CAD build for the part. Positions are in the model's coordinates, mm. A direction names the side the tool comes from. Coordinates: 2 decimals unless noted, no trailing zeros. Order: outer loops, then holes, each group sorted by start corner. A loop starts at its lowest first (then second) coordinate and runs counter-clockwise, first axis right, second up. Notation, with made-up numbers: (77.25, 0) - (130.25, 0) arc R21 cw to (130.25, 4) - close; hole circle Ø2 at (63.25, -33). An arc over 180 degrees is marked (long way). Write each question's results on one line, items separated by ' | '. Start each with the question number.
Q1. Band-saw the part on B-B, the plane z = 28.5. Write the cut outline in (x, y).
Q2. Band-saw the part on A-A, the plane x = -49. Write the cut outline in (y, z).
Q3. Band-saw the part on D-D, the plane z = -6. Write the cut outline in (x, y), then the cut area to 3 significant figures.
Q4. Wall check: probe 1 along X at (y, z) = (-11.5, -30.5); probe 2 along X at (y, z) = (40.5, 32.5); probe 3 along Z at (x, y) = (-5.5, 59). Give the ranges that are in metal, low to high.
Q5. Pin check, flat tips, straight feed: P1, Ø10, axis at x = 57.5, y = -5.5, coming from the +Z side; P2, Ø7.5, axis at y = 5, z = -31, coming from the +X side; P3, Ø12, axis at x = -0.5, y = 25.5, coming from the +Z side. Stop position of each tip, or through.
Q6. Band-saw the part on C-C, the plane z = 14. Write the cut outline in (x, y), then the cut area to 3 significant figures.
Q7. Which spindle directions (+Z, -Z, +X, -X, +Y, -Y) get a long thin tool onto all of the face, cutting with end or side? Do faces 1 (the flat face through (29.781, 1, -28)), 2 (the flat face through (46.28, 1.3, 44.5)), 3 (the flat face through (28.229, 1.301, 21.824)). Say none if no direction does.
Q8. Pull direction Z, two halves, no side cores. Call faces 4 (the flat face through (-46.28, 1.3, 44.5)), 5 (the flat face through (17.946, 1.301, -33.956)), 6 (the flat face through (1, 72.644, 3)), 7 (the flat face through (12.2, 1.3, 52.7)): released by +Z, released by -Z, zero draft, split by the parting line, or undercut.
```python
from build123d import *

# Parameters (mm, degrees)
F1_DEPTH      = 68.072
F1_DEPTH_BACK = 72.644


with BuildPart() as f1:
    # F0 (on Front) → F1 (new body, two sides)
    with BuildSketch(Plane.XZ) as f1_sk:
        with BuildLine():
            Line((-43.8699675724, 4.9395202659), (-26.3915906821, 9.9711745287))
            ThreePointArc((-26.3915906821, 9.9711745287), (-27.2085319986, 17.0209655839), (-26.1747674174, 24.042238818))
            Line((-26.1747674174, 24.042238818), (-30.3419636079, 19.5435739099))
            Line((-30.3419636079, 19.5435739099), (-43.8699675724, 4.9395202659))
        make_face()
        with BuildLine():
            ThreePointArc((-9.5438323287, 42.0849398232), (-15.4092627723, 39.0301381471), (-20.3645734785, 34.6506423572))
            Line((-20.3645734785, 34.6506423572), (-7.1865939535, 29.6427810635))
            Line((-7.1865939535, 29.6427810635), (-7.1865939535, 32.6668713242))
            Line((-7.1865939535, 32.6668713242), (-9.5438323287, 42.0849398232))
        make_face()
        with BuildLine():
            Line((0, -36.5192646342), (0, -10.610057041))
            ThreePointArc((0, -10.610057041), (-16.7339710743, -4.8564916944), (-26.3915906821, 9.9711745287))
            Line((-26.3915906821, 9.9711745287), (-43.8699675724, 4.9395202659))
            Line((-43.8699675724, 4.9395202659), (-30.3419636079, 19.5435739099))
            Line((-30.3419636079, 19.5435739099), (-65.5041635036, 38.4049154818))
            Line((-65.5041635036, 38.4049154818), (-60.6228390417, 21.448736815))
            Line((-60.6228390417, 21.448736815), (-43.8699675724, -2.8352683876))
            Line((-43.8699675724, -2.8352683876), (-40.2366704703, -3.5186973045))
            Line((-40.2366704703, -3.5186973045), (-43.8699675724, -9.0736041914))
            Line((-43.8699675724, -9.0736041914), (-37.7853512764, -20.751086995))
            Line((-37.7853512764, -20.751086995), (-29.7805646327, -25.9867765768))
            Line((-29.7805646327, -25.9867765768), (-29.7805646327, -29.878012836))
            Line((-29.7805646327, -29.878012836), (-25.9352512658, -32.3328636587))
            Line((-25.9352512658, -32.3328636587), (-21.6632075608, -32.3328636587))
            Line((-21.6632075608, -32.3328636587), (-14.1229508445, -35.6245934963))
            Line((-14.1229508445, -35.6245934963), (-14.1229508445, -25.9867765768))
            Line((-14.1229508445, -25.9867765768), (-8.1736836948, -29.878012836))
            Line((-8.1736836948, -29.878012836), (-3.4166643449, -34.2845275061))
            Line((-3.4166643449, -34.2845275061), (0, -36.5192646342))
        make_face()
        Polygon((0, 26.9117504358), (-7.1865939535, 29.6427810635), (-7.1865939535, 21.905059882), align=None)
        with BuildLine():
            Line((-7.1865939535, 42.5278679195), (-7.293939468, 42.8177008727))
            ThreePointArc((-7.293939468, 42.8177008727), (-8.4268543632, 42.4757869761), (-9.5438323287, 42.0849398232))
            Line((-9.5438323287, 42.0849398232), (-7.1865939535, 32.6668713242))
            Line((-7.1865939535, 32.6668713242), (-7.1865939535, 42.5278679195))
        make_face()
        with BuildLine():
            ThreePointArc((-20.3645734785, 34.6506423572), (-23.8665481201, 29.673348875), (-26.1747674174, 24.042238818))
            Line((-26.1747674174, 24.042238818), (-14.7990193218, 16.6017049924))
            Line((-14.7990193218, 16.6017049924), (-7.1865939535, 21.905059882))
            Line((-7.1865939535, 21.905059882), (-7.1865939535, 29.6427810635))
            Line((-7.1865939535, 29.6427810635), (-20.3645734785, 34.6506423572))
        make_face()
        with BuildLine():
            Line((-72.940915823, 54.6305663884), (-26.1747674174, 24.042238818))
            ThreePointArc((-26.1747674174, 24.042238818), (-23.8665481201, 29.673348875), (-20.3645734785, 34.6506423572))
            Line((-20.3645734785, 34.6506423572), (-72.940915823, 54.6305663884))
        make_face()
        with BuildLine():
            ThreePointArc((-26.1747674174, 24.042238818), (-27.2085319986, 17.0209655839), (-26.3915906821, 9.9711745287))
            Line((-26.3915906821, 9.9711745287), (-21.5597059578, 11.3621717319))
            Line((-21.5597059578, 11.3621717319), (-26.1747674174, 24.042238818))
        make_face()
        with BuildLine():
            ThreePointArc((-9.5438323287, 42.0849398232), (-8.4268543632, 42.4757869761), (-7.293939468, 42.8177008727))
            Line((-7.293939468, 42.8177008727), (-14.7990193218, 63.081420958))
            Line((-14.7990193218, 63.081420958), (-9.5438323287, 42.0849398232))
        make_face()
        Polygon((-4.6579921618, 35.7006415725), (-7.1865939535, 42.5278679195), (-7.1865939535, 32.6668713242), align=None)
        with BuildLine():
            Line((-7.1865939535, 42.5278679195), (-7.1865939535, 42.8473305385))
            ThreePointArc((-7.1865939535, 42.8473305385), (-7.2402818676, 42.8325706174), (-7.293939468, 42.8177008727))
            Line((-7.293939468, 42.8177008727), (-7.1865939535, 42.5278679195))
        make_face()
        with BuildLine():
            ThreePointArc((-26.3915906821, 9.9711745287), (-16.7339710743, -4.8564916944), (0, -10.610057041))
            ThreePointArc((0, -10.610057041), (19.2416214619, -2.6399164695), (27.2117620334, 16.6017049924))
            ThreePointArc((27.2117620334, 16.6017049924), (21.7356187496, 32.9737198511), (7.5112464838, 42.7562680593))
            Line((7.5112464838, 42.7562680593), (7.5112464838, 11.7172822356))
            Line((7.5112464838, 11.7172822356), (-7.1865939535, 11.7172822356))
            Line((-7.1865939535, 11.7172822356), (-7.1865939535, 21.905059882))
            Line((-7.1865939535, 21.905059882), (-14.7990193218, 16.6017049924))
            Line((-14.7990193218, 16.6017049924), (-26.1747674174, 24.042238818))
            Line((-26.1747674174, 24.042238818), (-21.5597059578, 11.3621717319))
            Line((-21.5597059578, 11.3621717319), (-26.3915906821, 9.9711745287))
        make_face()
        with BuildLine():
            Line((7.5112464838, 11.7172822356), (7.5112464838, 42.7562680593))
            ThreePointArc((7.5112464838, 42.7562680593), (0.1685909551, 43.8129447666), (-7.1865939535, 42.8473305385))
            Line((-7.1865939535, 42.8473305385), (-7.1865939535, 42.5278679195))
            Line((-7.1865939535, 42.5278679195), (-4.6579921618, 35.7006415725))
            Line((-4.6579921618, 35.7006415725), (-7.1865939535, 32.6668713242))
            Line((-7.1865939535, 32.6668713242), (-7.1865939535, 29.6427810635))
            Line((-7.1865939535, 29.6427810635), (0, 26.9117504358))
            Line((0, 26.9117504358), (-7.1865939535, 21.905059882))
            Line((-7.1865939535, 21.905059882), (-7.1865939535, 11.7172822356))
            Line((-7.1865939535, 11.7172822356), (7.5112464838, 11.7172822356))
        make_face()
        with BuildLine():
            ThreePointArc((-7.1865939535, 42.8473305385), (0.1685909551, 43.8129447666), (7.5112464838, 42.7562680593))
            Line((7.5112464838, 42.7562680593), (7.5112464838, 53.6164604127))
            Line((7.5112464838, 53.6164604127), (-7.1865939535, 53.6164604127))
            Line((-7.1865939535, 53.6164604127), (-7.1865939535, 42.8473305385))
        make_face()
    extrude(amount=F1_DEPTH)
    extrude(f1_sk.sketch, amount=-F1_DEPTH_BACK)

    # F2: F1 across plane


with BuildPart() as f1_1:
    add(f1.part)
    add(f1.part.mirror(Plane.YZ))


solid = f1_1.part
```
Results below:
1) outline: (-62.65, -68.07) - (-47.04, -68.07) - (-47.04, 72.64) - (-62.65, 72.64) - close; (-32.99, -68.07) - (32.99, -68.07) - (32.99, 72.64) - (-32.99, 72.64) - close; (47.04, -68.07) - (62.65, -68.07) - (62.65, 72.64) - (47.04, 72.64) - close
2) outline: (-68.07, 4.6) - (72.64, 4.6) - (72.64, 29.55) - (-68.07, 29.55) - close; (-68.07, 38.97) - (72.64, 38.97) - (72.64, 45.53) - (-68.07, 45.53) - close
3) outline: (-41.86, -68.07) - (41.86, -68.07) - (41.86, 72.64) - (-41.86, 72.64) - close | area: 11,800 mm²
4) probe 1: x = -28.81 to -14.12, -7.5 to 7.5, 14.12 to 28.81 | probe 2: x = -63.8 to -54.5, -39.11 to 39.11, 54.5 to 63.8 | probe 3: z = -32.35 to 53.62
5) P1: stops at z = 50.66 | P2: stops at x = 29.78 | P3: stops at z = 53.62
6) outline: (-55.48, -68.07) - (55.48, -68.07) - (55.48, 72.64) - (-55.48, 72.64) - close | area: 15,600 mm²
7) face 1: -Z, +X, +Y, -Y | face 2: +Z, +Y, -Y | face 3: +Y, -Y
8) face 4: released by +Z | face 5: released by -Z | face 6: zero draft | face 7: undercut
